Could you check a few things on this model? Use its own coordinates, in mm. A direction names the side the tool comes from. Round coordinates to 2 decimals unless told otherwise and drop trailing zeros. Write each loop counter-clockwise with the first axis right and the second up, starting at its lowest first coordinate (ties: lowest second). Pieces come first, ordered by that corner, then holes. Notation, with made-up numbers: (40.5, -5) - (93.5, -5) arc R21 ccw to (93.5, 17) - close; hole circle Ø6 at (62.5, 5). An arc over 180 degrees is marked (long way). Put each result on its own line as item: value.
Autodesk Inventor part; units mm, degrees
ref_plane "YZ Plane" through (0, 0, 0) normal (1, 0, 0) x (0, 1, 0)
ref_plane "XZ Plane" through (0, 0, 0) normal (0, 1, 0) x (-1, 0, 0)
ref_plane "XY Plane" through (0, 0, 0) normal (0, 0, 1) x (1, 0, 0)
sketch "Sketch1" plane through (0, 0, 0) normal (0, 1, 0) x (-1, 0, 0)
  line L0 (0, 0) -> (25, 0)
  line L1 (25, 0) -> (25, 52)
  line L2 (25, 52) -> (0, 52)
  line L3 (0, 52) -> (0, 42)
  line L4 (0, 0) -> (0, 10)
  arc A0 (0, 10) -> (0, 42) centre (0, 26) ccw
  dimension "d0" = 25
  dimension "d1" = 52
  dimension "d3" = 10
  dimension "d4" = 10
  dimension "d5" = 16
extrude "Extrusion1" add sketch "Sketch1" along normal blind 26
sketch "Sketch2" plane through (-25, 0, 0) normal (-1, 0, 0) x (0, 0, 1)
  line L0 (0, 26) -> (0, -19)
  line L1 (0, -19) -> (52, -19)
  line L2 (52, -19) -> (52, -9)
  line L3 (0, 26) -> (16, 26)
  line L4 (0, 26) -> (52, 26)
  arc A0 (16, 26) -> (52, -9) centre (55.7076, 30.8278) ccw
  point P0 (0, 0)
  dimension "d8" = 45
  dimension "d9" = 52
  dimension "d10" = 90
  dimension "d11" = 10
  dimension "d12" = 90
  dimension "d13" = 16
  dimension "d17" = 40
extrude "Extrusion2" add sketch "Sketch2" along normal blind 35
sketch "Sketch3" plane through (0, 0, 0) normal (0, -1, 0) x (1, 0, 0)
  line L0 (-25, 0) -> (-25, 30.2194)
  line L1 (-25, 0) -> (10, 0)
  line L2 (10, 52) -> (-25, 52)
  line L3 (-25, 52) -> (-25, 0)
  line L4 (10, 0) -> (10, 16)
  line L5 (10, 52) -> (10, 36)
  line L6 (10, 16) -> (15, 16)
  line L7 (15, 16) -> (15, 36)
  line L8 (15, 36) -> (10, 36)
  line L9 (10, 36) -> (10, 16)
  point P0 (0, 0)
  point P1 (10, 36)
  dimension "d18" = 35
  dimension "d19" = 16
  dimension "d20" = 16
  dimension "d21" = 5
  dimension "d27" = 35
extrude "Extrusion3" add sketch "Sketch3" along normal blind 19
sketch "Sketch4" plane through (10, 0, 36) normal (0, 0, 1) x (1, 0, 0)
  line L0 (5, 0) -> (5, -19)
  line L1 (5, -19) -> (17, -19)
  line L2 (17, -19) -> (5, 0)
  line L3 (5, 0) -> (5, -19)
  point P0 (-10, 0)
  dimension "d24" = 12
extrude "Extrusion4" add sketch "Sketch4" against normal blind 20
equation "\"d20\" = d19"
equation "\"d27\" = d18"
(1) For faces 1 (the face through (10, -9, 8)), 2 (the face through (16, -11, 36)), 3 (the face through (0, 13, 47)), which set-ups out of +Z, -Z, +X, -X, +Y, -Y let a thin tool reach every point of the face, with its end or its side?
Values found:
face 1: -Z, +X, +Y, -Y
face 2: +Z, +X, +Y, -Y
face 3: +Z, -Z, +X, +Y
(2) Please list where these lines run through material, in increasing order: probe 1 along X at (y, z) = (11.5, 46.5); probe 2 along X at (y, z) = (-5.5, 48.5); probe 3 along Y at (x, z) = (-4.5, 16). Write a range as from..to.
Values found:
probe 1: x = -25..0
probe 2: x = -25..10
probe 3: y = -19..0
(3) If we mould it in two halves opening along Z, with no side actions, what happens to faces 4 (the face through (16, -11, 16)), 5 (the face through (0, 13, 5)), 6 (the face through (3, 0, 26)), 7 (the face through (-16, 13, 26))? For each: pulls with the +Z half, pulls with the -Z half, needs draft (parallel to the pull), parting line crosses it, or undercut.
Values found:
face 4: pulls with the -Z half
face 5: needs draft
face 6: undercut
face 7: undercut
(4) Imagine slicing it at D-D, the plane x = 21. List the corners of the cut face in (y, z) for me, then the cut area to 3 significant figures.
Values found:
outline: (-19, 16) - (-9.5, 16) - (-9.5, 36) - (-19, 36) - close
area: 190 mm^2
(5) Imagine slicing it at B-B, the plane y = 19.5. List the corners of the cut face in (x, z) for me.
Values found:
outline: (-60, 0) - (0, 0) - (0, 10) arc R16 cw to (0, 42) - (0, 52) - (-25, 52) - (-25, 17.35) - (-60, 17.35) - close
(6) Imagine slicing it at C-C, the plane x = -31.5. List the corners of the cut face in (y, z) for me.
Values found:
outline: (-19, 0) - (26, 0) - (26, 16) arc R40 cw to (-9, 52) - (-19, 52) - close
(7) I'm going to push flat-ended pins straight in: pin 1 (8 mm diameter, centred on y = 13.5, z = 47, fed in from +X); pin 2 (13.5 mm diameter, centred on x = 17, y = -8.5, fed in from +Z); pin 3 (1.5 mm diameter, centred on x = -44, y = 6, fed in from +Z); pin 4 (6 mm diameter, centred on x = -27.5, y = -2, fed in from -Z). Where does each tip first touch, or does it pass through?
Values found:
pin 1: stops at x = 0
pin 2: stops at z = 36
pin 3: stops at z = 24.95
pin 4: stops at z = 0
(8) Imagine slicing it at A-A, the plane z = 47. List the corners of the cut face in (x, y) for me, then the cut area to 3 significant figures.
Values found:
outline: (-60, -19) - (10, -19) - (10, 0) - (0, 0) - (0, 26) - (-25, 26) - (-25, -8.21) - (-60, -8.21) - close
area: 1,690 mm^2
